```python
from build123d import *

# Parameters (mm, degrees)
SKETCH1_W           = 300
SKETCH1_H           = 300
BOSS_EXTRUDE1_DEPTH = 32
SKETCH2_W           = 300
SKETCH2_H           = 120
BOSS_EXTRUDE2_DEPTH = 28
SKETCH3_W           = 120
SKETCH3_H           = 70
BOSS_EXTRUDE3_DEPTH = 80
CUT_EXTRUDE1_DEPTH  = 120


with BuildPart() as part:
    # Sketch1 → Boss-Extrude1 (new body)
    with BuildSketch(Plane(origin=(0, 0, 0), x_dir=(1, 0, 0), z_dir=(0, 1, 0))):
        Rectangle(SKETCH1_W, SKETCH1_H)
    extrude(amount=BOSS_EXTRUDE1_DEPTH)

    # Sketch2 → Boss-Extrude2 (add)
    with BuildSketch(Plane(origin=(0, 32, 0), x_dir=(1, 0, 0), z_dir=(0, 1, 0))):
        with Locations((0, 40)):
            Rectangle(SKETCH2_W, SKETCH2_H)
    extrude(amount=BOSS_EXTRUDE2_DEPTH)

    # Sketch3 → Boss-Extrude3 (add)
    with BuildSketch(Plane(origin=(0, 32, 0), x_dir=(1, 0, 0), z_dir=(0, 1, 0))):
        with Locations((0, -115)):
            Rectangle(SKETCH3_W, SKETCH3_H)
    extrude(amount=BOSS_EXTRUDE3_DEPTH)

    # Sketch4 → Cut-Extrude1 (cut)
    with BuildSketch(Plane(origin=(60, 0, 0), x_dir=(0, 0, -1), z_dir=(1, 0, 0))):
        Polygon((-80, 112), (-150, 42), (-150, 112), align=None)
    extrude(amount=-CUT_EXTRUDE1_DEPTH, mode=Mode.SUBTRACT)


solid = part.part
```
Geometry: final body of the model. Coordinates: model frame, mm. A direction names the side the tool comes from. Give positions to 0.01 mm unless a question says otherwise; leave off trailing zeros. Order: outer loops, then holes, each group sorted by start corner. A loop starts at its lowest first (then second) coordinate and runs counter-clockwise, first axis right, second up. Notation, with made-up numbers: (24.25, 27.5) -> (71.25, 27.5) arc R20 ccw to (71.25, 33.5) -> close; hole circle Ø6 at (84.25, -25). An arc over 180 degrees is marked (long way). Write each question's results on one line, items separated by ' | '. Start each with the question number.
1) Draft query along Z for faces 6 (the flat face through (-2, 46, 20)), 7 (the flat face through (-2, 16, -150)), 8 (the flat face through (-2, 0, -2)). Return one class per face: pulls with the +Z half, pulls with the -Z half, needs draft (parallel to the pull), parting line crosses it, or undercut.
2) Line query: line 1 (Z direction, x = 45.5, y = 36); line 2 (Y direction, x = 47.5, z = -28); line 3 (Z direction, x = 128, y = 37). Output: solid intervals per line, ascending. Write a range as from..to.
3) Section D-D (x = -94.5). Return loops of the section in (y, z), then the cut area to 3 significant figures.
4) Section A-A (z = 114.5). Return loops of the section in (x, y).
5) Section B-B (x = 12.5). Return loops of the section in (y, z).
6) Section C-C (y = 91). Return loops of the section in (x, z).
7) Set-up query: faces 1 (the flat face through (60, 63, 108)), 2 (the flat face through (-2, 46, -100)), 3 (the flat face through (-60, 63, 108)), 4 (the flat face through (-150, 23, 2)), 5 (the flat face through (-1, 71, 80)). Return all of +Z, -Z, +X, -X, +Y, -Y with unobstructed straight access to the full face (end or side cutting, diameter ignored); none if empty.
8) First-contact query: pin 1 (2 mm diameter, centred on x = 86, z = 120, fed in from +Y); pin 2 (12 mm diameter, centred on x = 67, z = -24.5, fed in from +Y); pin 3 (21 mm diameter, centred on y = 66.5, z = 124.5, fed in from +X). Flat tips, straight axial feed; report the tip coordinate or a pass-through.
Calculated:
1) face 6: undercut | face 7: pulls with the -Z half | face 8: needs draft
2) line 1: -100..20, 80..150 | line 2: 0..60 | line 3: -100..20
3) outline: (0, -150) -> (32, -150) -> (32, -100) -> (60, -100) -> (60, 20) -> (32, 20) -> (32, 150) -> (0, 150) -> close | area: 13,000 mm2
4) outline: (-150, 0) -> (150, 0) -> (150, 32) -> (60, 32) -> (60, 77.5) -> (-60, 77.5) -> (-60, 32) -> (-150, 32) -> close
5) outline: (0, -150) -> (32, -150) -> (32, -100) -> (60, -100) -> (60, 20) -> (32, 20) -> (32, 80) -> (112, 80) -> (42, 150) -> (0, 150) -> close
6) outline: (-60, 80) -> (60, 80) -> (60, 101) -> (-60, 101) -> close
7) face 1: +Z, +X, +Y | face 2: -Z, +X, -X, +Y | face 3: +Z, -X, +Y | face 4: +Z, -Z, -X, +Y, -Y | face 5: +X, -X, +Y
8) pin 1: y = 32 | pin 2: y = 60 | pin 3: x = 60
